The model under review builds one solid part; all positions refer to its coordinate system, in mm. Round coordinates to 2 decimals unless told otherwise and drop trailing zeros. Loops run counter-clockwise (first coordinate to the right, second up) from the corner with the lowest first, then second, coordinate; pieces in that order, holes last. Notation, with made-up numbers: M 44.5,57.5 L 70.5,57.5 A11 ccw 70.5,76.5 Z; hole C -13,74 d11. An arc over 180 degrees is marked long. Answer as a JSON object with one key per item and string values. Group by question number.
Item 1: Insertion check: P1, Ø9.5, axis at x = 17.96, z = -17.96, coming from the -Y side; P2, Ø10, axis at x = 0, z = 0, coming from the +Y side; P3, Ø3.5, axis at x = 16, z = 20.5, coming from the +Y side. Each pin has a flat end and moves straight along its axis. Give the tip position at first contact, or say it passes through.
Item 2: Consider section B-B (x = 0). Give the boundary of the cut face in (y, z).
Item 3: To check wall thickness, follow line 1 (X direction, y = 0, z = -18); line 2 (Z direction, x = -16.5, y = -1.1); line 3 (X direction, y = -1.1, z = -20.5). State the ranges of each line that lie inside material, in increasing order.
Item 4: Consider section C-C (x = -16). Give the boundary of the cut face in (y, z), and give its area (3 significant figures).
Item 5: Consider section A-A (z = 0). Give the boundary of the cut face in (x, y), and give its area (3 significant figures).
Item 6: Consider section D-D (y = 0.2). Give the boundary of the cut face in (x, z) (3 decimals), and give its area (3 significant figures).
```python
from build123d import *

# Parameters (mm, degrees)
SKETCH2_R                   = 39.2557
BOSS_EXTRUDE1_DEPTH         = 1.5875
F_1_4_0_25_DIAMETER_HOLE1_D = 6.35
F_1_2_0_5_DIAMETER_HOLE1_D  = 12.7
SKETCH10_R                  = 6.0325
CUT_EXTRUDE1_DEPTH          = 0.79375


with BuildPart() as part:
    # Sketch2 → Boss-Extrude1 (new body, symmetric)
    with BuildSketch(Plane(origin=(0, 0, 0), x_dir=(1, 0, 0), z_dir=(0, 1, 0))):
        Circle(SKETCH2_R)
    extrude(amount=BOSS_EXTRUDE1_DEPTH, both=True)

    # 1/4 (0.25) Diameter Hole1 (through all)
    with Locations(Plane(origin=(0, 1.5875, 0), x_dir=(1, 0, 0), z_dir=(0, 1, 0))):
        with Locations((-17.960512242, -17.960512242), (-17.960512242, 17.960512242), (17.960512242, 17.960512242), (17.960512242, -17.960512242)):
            Hole(F_1_4_0_25_DIAMETER_HOLE1_D / 2)

    # 1/2 (0.5) Diameter Hole1 (through all)
    with Locations(Plane(origin=(0, 1.5875, 0), x_dir=(1, 0, 0), z_dir=(0, 1, 0))):
        with Locations((0, 0)):
            Hole(F_1_2_0_5_DIAMETER_HOLE1_D / 2)

    # Sketch10 → Cut-Extrude1 (cut)
    with BuildSketch(Plane(origin=(0, 1.5875, 0), x_dir=(1, 0, 0), z_dir=(0, 1, 0))):
        with Locations((-17.960512242, 17.960512242)):
            Circle(SKETCH10_R)
        with Locations((17.960512242, 17.960512242)):
            Circle(SKETCH10_R)
        with Locations((17.960512242, -17.960512242)):
            Circle(SKETCH10_R)
        with Locations((-17.960512242, -17.960512242)):
            Circle(SKETCH10_R)
    cut_extrude1 = extrude(amount=-CUT_EXTRUDE1_DEPTH, mode=Mode.SUBTRACT)

    # Mirror1: Cut-Extrude1 across plane
    add(cut_extrude1.mirror(Plane.ZX), mode=Mode.SUBTRACT)


solid = part.part
```
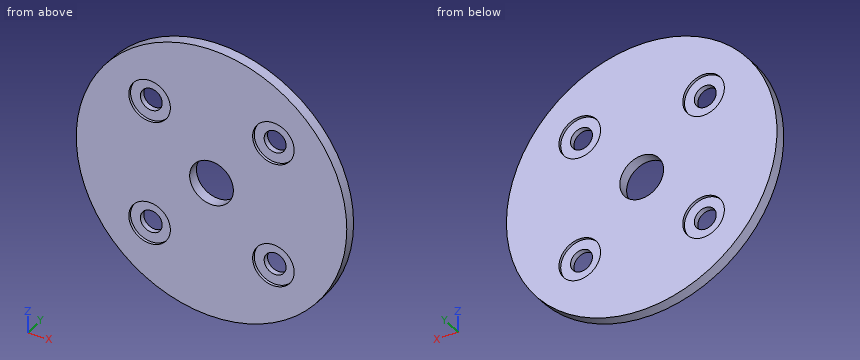
Geometry results:
{
 "1": {"P1": "stops at y = -0.79", "P2": "passes through", "P3": "stops at y = 0.79"},
 "2": {"outline": "M -1.59,-39.26 L 1.59,-39.26 L 1.59,-6.35 L -1.59,-6.35 Z; M -1.59,6.35 L 1.59,6.35 L 1.59,39.26 L -1.59,39.26 Z"},
 "3": {"line 1": "x = -34.89 to -21.14, -14.79 to 14.79, 21.14 to 34.89", "line 2": "z = -35.62 to -23.81, -12.11 to 12.11, 23.81 to 35.62", "line 3": "x = -33.48 to -23.43, -12.49 to 12.49, 23.43 to 33.48"},
 "4": {"outline": "M -1.59,-35.85 L 1.59,-35.85 L 1.59,-23.67 L 0.79,-23.67 L 0.79,-20.46 L -0.79,-20.46 L -0.79,-23.67 L -1.59,-23.67 Z; M -1.59,-12.26 L -0.79,-12.26 L -0.79,-15.46 L 0.79,-15.46 L 0.79,-12.26 L 1.59,-12.26 L 1.59,12.26 L 0.79,12.26 L 0.79,15.46 L -0.79,15.46 L -0.79,12.26 L -1.59,12.26 Z; M -1.59,23.67 L -0.79,23.67 L -0.79,20.46 L 0.79,20.46 L 0.79,23.67 L 1.59,23.67 L 1.59,35.85 L -1.59,35.85 Z", "area": "176 mm^2"},
 "5": {"outline": "M -39.26,-1.59 L -6.35,-1.59 L -6.35,1.59 L -39.26,1.59 Z; M 6.35,-1.59 L 39.26,-1.59 L 39.26,1.59 L 6.35,1.59 Z", "area": "209 mm^2"},
 "6": {"outline": "C 0,0 d78.511; hole C -17.961,-17.961 d6.35; hole C -17.961,17.961 d6.35; hole C 0,0 d12.7; hole C 17.961,-17.961 d6.35; hole C 17.961,17.961 d6.35", "area": "4,590 mm^2"}
}
